Verification items for the finished model (mm, model axes). Face numbers are marked on the shaded views. A direction names the side the tool comes from. Round coordinates to 2 decimals unless told otherwise and drop trailing zeros. Loops run counter-clockwise (first coordinate to the right, second up) from the corner with the lowest first, then second, coordinate; pieces in that order, holes last. Notation, with made-up numbers: (-24, 71.25) -> (11, 71.25) arc R35 cw to (11, 107.25) -> close; hole circle Ø6 at (-1, 82). An arc over 180 degrees is marked (long way). Use CSV: the item, a comma, the result in double quotes. Start each with the question number.
Autodesk Inventor part; units mm, degrees
ref_plane "p1_XY" through (0, 0, 0) normal (0, 1, 0) x (1, 0, 0)
ref_plane "p1_YZ" through (0, 0, 0) normal (1, 0, 0) x (0, 0, -1)
ref_plane "p1_ZX" through (0, 0, 0) normal (0, 0, -1) x (0, 1, 0)
sketch "Sketch_1" plane through (0, 0, 0) normal (0, 0, 1) x (1, 0, 0)
  line L0 (-9, 6.5) -> (-9, 0)
  line L1 (-9, 0) -> (9, 0)
  line L2 (9, 0) -> (9, 6.5)
  line L3 (9, 6.5) -> (7.1, 6.5)
  line L4 (7.1, 6.5) -> (7.1, 8.4)
  line L5 (7.1, 8.4) -> (-7.1, 8.4)
  line L6 (-7.1, 8.4) -> (-7.1, 6.5)
  line L7 (-7.1, 6.5) -> (-9, 6.5)
extrude "Extrusion1" add sketch "Sketch_1" along normal mid plane 8.2
ref_plane "p1_XY" through (0, 0, 0) normal (0, 1, 0) x (1, 0, 0)
ref_plane "p1_YZ" through (0, 0, 0) normal (1, 0, 0) x (0, 0, -1)
ref_plane "p1_ZX" through (0, 0, 0) normal (0, 0, -1) x (0, 1, 0)
properties part number "GUS Zentriereinsatz"
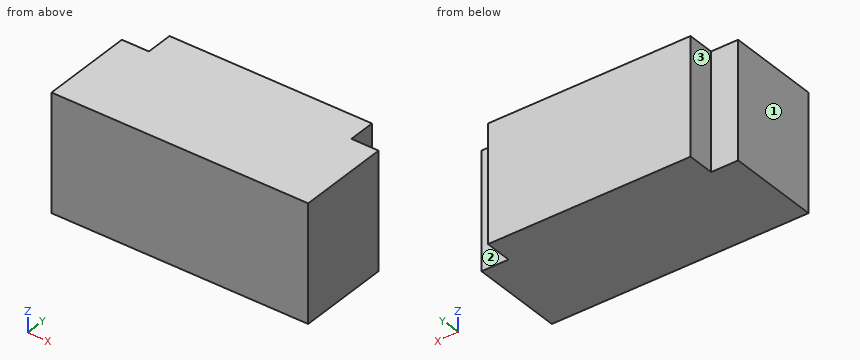
Q1. Tool access check on the marked faces 1, 2 and 3. Record the directions out of +Z, -Z, +X, -X, +Y, -Y that give a thin tool (end or side, any length) a straight path to the whole face; none if there is none.
Q2. Thickness scan on L1, parallel to Y at x = 7.25, z = 2.5; L2, parallel to X at y = 7.25, z = 0.25. Record the ranges inside material, lowest first. Write a range as from..to.
Q3. Cross-section at A-A (z = 0). Record the boundary of the cut face in (x, y).
Q4. Depth check by flat-ended pin: pin 1 Ø0.6 at (y, z) = (7, -1.5) entering from +X; pin 2 Ø0.6 at (y, z) = (7, -0.5) entering from -X. Enter the tip coordinate at first touch or a pass-through.
Answer list:
1,face 1,"+Z, -Z, -X, +Y, -Y"
1,face 2,"+Z, -Z, +X, +Y"
1,face 3,"+Z, -Z, -X, +Y"
2,L1,"y = 0..6.5"
2,L2,"x = -7.1..7.1"
3,outline,"(-9, 0) -> (9, 0) -> (9, 6.5) -> (7.1, 6.5) -> (7.1, 8.4) -> (-7.1, 8.4) -> (-7.1, 6.5) -> (-9, 6.5) -> close"
4,pin 1,"stops at x = 7.1"
4,pin 2,"stops at x = -7.1"
